Here's how the part is built. I have some questions about the finished solid (model axes, mm). Coordinates: 2 decimals unless noted, no trailing zeros. Write each loop counter-clockwise with the first axis right and the second up, starting at its lowest first coordinate (ties: lowest second). Pieces come first, ordered by that corner, then holes. Notation, with made-up numbers: M 77.5,-5 L 114.5,-5 A29 cw 114.5,16 Z; hole C -6,82.25 d11. An arc over 180 degrees is marked long. Use one line per item in the form item = value. Start each with the question number.
1. I want a section at B-B, the plane y = 0. List the corners of the cut face in (x, z) for me, plus the area to 3 significant figures.
2. Please list where these lines run through material, in increasing order: line 1 along Z through (x, y) = (-12.5, -17.6); line 2 along X through (y, z) = (-17.5, 150); line 3 along Y through (x, z) = (13.5, 165.5). Write a range as [from, to].
3. I want a section at C-C, the plane x = 0. List the corners of the cut face in (y, z) for me, plus the area to 3 significant figures.
4. I'm going to push flat-ended pins straight in: pin 1 Ø5 at (y, z) = (-12, 202.5) entering from -X; pin 2 Ø1.6 at (y, z) = (-13.5, 188) entering from +X; pin 3 Ø3.5 at (x, z) = (-12.5, 250) entering from +Y; pin 4 Ø10.5 at (x, z) = (13.5, 176.5) entering from +Y. Where does each tip first touch, or does it pass through?
Autodesk Inventor part; units mm, degrees
ref_plane "YZ Plane" through (0, 0, 0) normal (1, 0, 0) x (0, 1, 0)
ref_plane "XZ Plane" through (0, 0, 0) normal (0, 1, 0) x (-1, 0, 0)
ref_plane "XY Plane" through (0, 0, 0) normal (0, 0, 1) x (1, 0, 0)
sketch "Sketch1" plane through (0, 0, 0) normal (0, 0, 1) x (1, 0, 0)
  circle A0 centre (0, 0) radius 6
  line L0 (-3, -5.1962) -> (-6.0022, -10.3962)
  line L1 (-6.0022, -10.3962) -> (6.0022, -10.3962)
  line L2 (6.0022, -10.3962) -> (3, -5.1962)
  line L3 (-7.5, -20.1962) -> (7.5, -20.1962)
  line L4 (7.5, -20.1962) -> (7.5, -10.3962)
  line L5 (7.5, -10.3962) -> (-7.5, -10.3962)
  line L6 (-7.5, -10.3962) -> (-7.5, -20.1962)
  line L7 (0, -10.3962) -> (0, 0)
  line L8 (-17, -15.6962) -> (17, -15.6962)
  line L9 (17, -15.6962) -> (17, -20.1962)
  line L10 (17, -20.1962) -> (-17, -20.1962)
  line L11 (-17, -20.1962) -> (-17, -15.6962)
  point P0 (0, -20.1962)
  dimension "d0" = 12
  dimension "d1" = 60
  dimension "d2" = 3
  dimension "d3" = 3
  dimension "d4" = 15
  dimension "d5" = 9.8
  dimension "d6" = 15
  dimension "d7" = 4.5
  dimension "d8" = 34
extrude "Extrusion1" add sketch "Sketch1" along normal blind 300
sketch "Sketch2" plane through (0, 0, 300) normal (0, 0, 1) x (1, 0, 0)
  arc A0 (3, -5.1962) -> (-3, -5.1962) centre (0, 0) ccw
  line L0 (3, -5.1962) -> (6.0022, -10.3962)
  line L1 (6.0022, -10.3962) -> (7.5, -10.3962)
  line L2 (7.5, -10.3962) -> (7.5, -15.6962)
  line L3 (7.5, -15.6962) -> (17, -15.6962)
  line L4 (17, -15.6962) -> (17, -20.1962)
  line L5 (17, -20.1962) -> (-17, -20.1962)
  line L6 (-17, -20.1962) -> (-17, -15.6962)
  line L7 (-17, -15.6962) -> (-7.5, -15.6962)
  line L8 (-7.5, -15.6962) -> (-7.5, -10.3962)
  line L9 (-7.5, -10.3962) -> (-6.0022, -10.3962)
  line L10 (-6.0022, -10.3962) -> (-3, -5.1962)
  line L11 (-6, -19.1962) -> (6, -19.1962)
  line L12 (6, -19.1962) -> (6, -20.1962)
  line L13 (6, -20.1962) -> (-6, -20.1962)
  line L14 (-6, -20.1962) -> (-6, -19.1962)
  point P0 (0, -20.1962)
  dimension "d11" = 12
  dimension "d12" = 1
extrude "Extrusion2" cut sketch "Sketch2" against normal through all contours L5 L14 L11 L12
chamfer "Chamfer1" distance 1 angle 45 2 edges at (-6, -19.1962, 150) (6, -19.1962, 150)
sketch "Sketch3" plane through (-17, -20.1962, 0) normal (0, -1, 0) x (1, 0, 0)
  line L0 (23, 0) -> (23, 300) construction
  line L1 (23, 300) -> (34, 300)
  line L2 (34, 300) -> (34, 0)
  line L3 (34, 0) -> (23, 0) construction
  line L4 (11, 300) -> (11, 0) construction
  line L5 (11, 0) -> (0, 0) construction
  line L6 (0, 0) -> (0, 300)
  line L7 (0, 300) -> (11, 300)
  circle A0 centre (4.5, 50) radius 2
  circle A1 centre (29.5, 50) radius 2
  line L8 (29.5, 50) -> (4.5, 50) construction
  line L9 (17, 50) -> (17, 0) construction
  dimension "d18" = 50
  dimension "d19" = 4
  dimension "d20" = 4
  dimension "d21" = 25
extrude "Extrusion3" cut sketch "Sketch3" against normal through all
thread "Thread1"
thread "Thread2"
pattern_linear "Rectangular Pattern1" count 3 spacing 100 along (0, 0, 1) of "Extrusion3"
properties part number "sbr12_300mm"
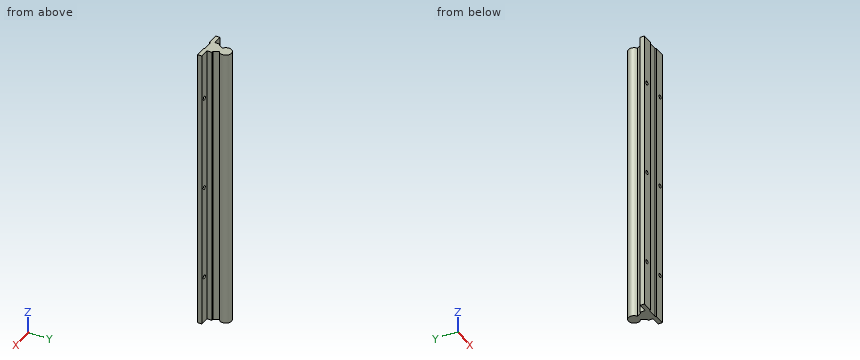
Answer list:
q1.outline = M -6,0 L 6,0 L 6,300 L -6,300 Z
q1.area = 3,600 mm²
q2.line_1 = [0, 48], [52, 148], [152, 248], [252, 300]
q2.line_2 = [-17, -14.5], [-10.5, 10.5], [14.5, 17]
q2.line_3 = [-20.2, -15.7]
q3.outline = M -19.2,0 L 6,0 L 6,300 L -19.2,300 Z
q3.area = 7,560 mm²
q4.pin_1 = -7.5
q4.pin_2 = 7.5
q4.pin_3 = through
q4.pin_4 = -15.7
